Here's how the part is built. I have some questions about the finished solid (model axes, mm). Face numbers are marked on the shaded views. A direction names the side the tool comes from. Round coordinates to 2 decimals unless told otherwise and drop trailing zeros. Write each loop counter-clockwise with the first axis right and the second up, starting at its lowest first coordinate (ties: lowest second). Pieces come first, ordered by that corner, then holes. Notation, with made-up numbers: (12.5, 36.25) - (46.5, 36.25) arc R23 ccw to (46.5, 68.25) - close; hole circle Ø2 at (-25.75, 86.25). An arc over 180 degrees is marked (long way). Return JSON: item names as keys, results as strings. Group by question number.
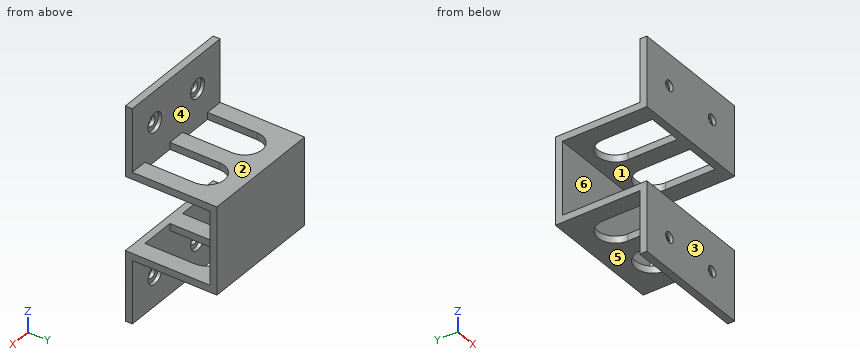
Autodesk Inventor part; units mm, degrees
ref_plane "YZ Plane" through (0, 0, 0) normal (1, 0, 0) x (0, 1, 0)
ref_plane "XZ Plane" through (0, 0, 0) normal (0, 1, 0) x (-1, 0, 0)
ref_plane "XY Plane" through (0, 0, 0) normal (0, 0, 1) x (1, 0, 0)
sketch "Sketch1" plane through (0, 0, 0) normal (0, 1, 0) x (-1, 0, 0)
  line L0 (0, 0) -> (-35, 0)
  line L1 (-35, 0) -> (-35, -20)
  line L2 (-35, -20) -> (0, -20)
  line L3 (0, -20) -> (0, 0)
  dimension "d0" = 35
  dimension "d1" = 20
extrude "Extrusion1" add sketch "Sketch1" along normal blind 2
sketch "Sketch2" plane through (0, 2, 0) normal (0, 1, 0) x (1, 0, 0)
  line L0 (0, 20) -> (0, 0)
  line L1 (35, 0) -> (35, 20)
  line L2 (0, 0) -> (35, 0)
  line L3 (35, 0) -> (35, 2)
  line L4 (35, 2) -> (0, 2)
  line L5 (0, 2) -> (0, 0)
  dimension "d4" = 2
extrude "Extrusion2" add sketch "Sketch2" along normal blind 24.2
sketch "Sketch3" plane through (0, 0, 0) normal (0, 0, 1) x (1, 0, 0)
  line L0 (0, 0) -> (0, 26.2)
  line L1 (35, 0) -> (35, 26.2)
  line L2 (0, 26.2) -> (35, 26.2)
  line L3 (35, 26.2) -> (35, 24.2)
  line L4 (35, 24.2) -> (0, 24.2)
  line L5 (0, 24.2) -> (0, 26.2)
  dimension "d7" = 2
extrude "Extrusion3" add sketch "Sketch3" along normal blind 23
sketch "Sketch4" plane through (0, 24.2, 0) normal (0, -1, 0) x (1, 0, 0)
  line L0 (35, -2) -> (35, 23)
  line L1 (0, 0) -> (0, 23)
  line L2 (35, 23) -> (0, 23)
  line L3 (0, 23) -> (0, 21)
  line L4 (0, 21) -> (35, 21)
  line L5 (35, 21) -> (35, 23)
  dimension "d10" = 2
extrude "Extrusion4" add sketch "Sketch4" along normal blind 24.2
sketch "Sketch5" plane through (0, 0, 23) normal (0, 0, 1) x (1, 0, 0)
  line L0 (0, 0) -> (0, 2)
  line L1 (35, 2) -> (0, 2)
  line L2 (0, 0) -> (35, 0)
  line L3 (35, 0) -> (35, 2)
  line L4 (35, 2) -> (0, 2)
  line L5 (0, 2) -> (0, 0)
extrude "Extrusion5" add sketch "Sketch5" along normal blind 18
sketch "Sketch6" plane through (0, 2, 0) normal (0, 1, 0) x (1, 0, 0)
  circle A0 centre (26, 11) radius 1.5
  line L0 (35, 20) -> (0, 20)
  line L1 (35, 2) -> (35, 20)
  circle A1 centre (9, 11) radius 1.5
  circle A2 centre (26, 11) radius 2.75
  circle A3 centre (9, 11) radius 2.75
  point P0 (0, 0)
  dimension "d15" = 3
  dimension "d16" = 9
  dimension "d17" = 9
  dimension "d18" = 3
  dimension "d19" = 17
  dimension "d20" = 5.5
  dimension "d21" = 5.5
extrude "Extrusion6" cut sketch "Sketch6" against normal blind 2 contours A0 | A1
extrude "Extrusion7" cut sketch "Sketch6" against normal blind 1
sketch "Sketch7" plane through (0, 2, 23) normal (0, 1, 0) x (1, 0, 0)
  circle A0 centre (26, -9) radius 1.5
  line L0 (35, -18) -> (0, -18)
  line L1 (35, 0) -> (35, -18)
  circle A1 centre (9, -9) radius 1.5
  circle A2 centre (26, -9) radius 2.75
  circle A3 centre (9, -9) radius 2.75
  point P0 (0, 23)
  dimension "d26" = 3
  dimension "d27" = 9
  dimension "d28" = 9
  dimension "d29" = 3
  dimension "d30" = 17
  dimension "d31" = 5.5
  dimension "d32" = 5.5
extrude "Extrusion8" cut sketch "Sketch7" against normal blind 2 contours A0 | A1
extrude "Extrusion9" cut sketch "Sketch7" against normal blind 1
sketch "Sketch8" plane through (35, 2, -2) normal (0, 0, -1) x (-1, 0, 0)
  arc A0 (15, 14.2) -> (5, 14.2) centre (10, 14.2) ccw
  line L0 (0, 24.2) -> (35, 24.2)
  line L1 (0, 0) -> (0, 24.2)
  line L2 (17.5, 24.2) -> (17.5, 0)
  line L3 (35, 0) -> (0, 0)
  line L4 (5, 14.2) -> (5, -0.3272)
  line L5 (15, 14.2) -> (15, 0)
  arc A1 (30, 14.2) -> (20, 14.2) centre (25, 14.2) ccw
  line L6 (30, 14.2) -> (30, -0.3272)
  line L7 (20, 14.2) -> (20, 0)
  point P0 (35, -2)
  point P1 (20, 0)
  point P2 (30, 0)
  point P3 (5, 0)
  dimension "d37" = 10
  dimension "d38" = 10
  dimension "d39" = 10
extrude "Extrusion10" cut sketch "Sketch8" against normal blind 25 contours L5 L3 L4 A0 | L7 A1 L6 L3
properties part number "Bracket Motor_3DPrint"
1) Will these pins go through, and if not, where does the flat tip stop? pin 1 Ø0.6 at (y, z) = (7, -1) entering from -X; pin 2 Ø1.6 at (x, z) = (8, -10) entering from +Y; pin 3 Ø4 at (x, z) = (30, 16) entering from -Y; pin 4 Ø12 at (x, y) = (19.5, 17) entering from -Z.
2) Imagine slicing it at D-D (x = 33.5). Please give me the cut outline in (y, z).
3) For the marked faces 1, 2 and 3, which set-ups out of +Z, -Z, +X, -X, +Y, -Y let a thin tool reach every point of the face, with its end or its side?
4) If we mould it in two halves opening along Z, with no side actions, what happens to the marked faces 4, 5 and 6? For each: released by +Z, released by -Z, zero draft, split by the parting line, or undercut.
5) I need wall thicknesses on line 1 along Z through (x, y) = (9, 1.4); line 2 along Z through (x, y) = (9, 0.4); line 3 along Y through (x, z) = (19, 1). Which ranges of each line are inside material? Lowest first, please.
6) Imagine slicing it at C-C (x = 26). Give the number of separate pieces and of enclosed holes in the cut face, plus the area to 3 significant figures.
7) Imagine slicing it at A-A (y = 14.5). Please give me the cut outline in (x, z), plus the area to 3 significant figures.
8) Imagine slicing it at B-B (z = -11). Please give me the cut outline in (x, y).
Results found:
{
 "1": {"pin 1": "stops at x = 0", "pin 2": "stops at y = 1", "pin 3": "stops at y = 24.2", "pin 4": "stops at z = -2"},
 "2": {"outline": "(0, -20) - (2, -20) - (2, -2) - (26.2, -2) - (26.2, 23) - (2, 23) - (2, 41) - (0, 41) - (0, 21) - (24.2, 21) - (24.2, 0) - (0, 0) - close"},
 "3": {"face 1": "+X, -X, -Y", "face 2": "+Z, +X, -X, +Y", "face 3": "+Z, -Z, +X, -X, -Y"},
 "4": {"face 4": "zero draft", "face 5": "released by -Z", "face 6": "undercut"},
 "5": {"line 1": "z = -20 to -13.75, -8.25 to 0, 21 to 29.25, 34.75 to 41", "line 2": "z = -20 to -12.5, -9.5 to 0, 21 to 30.5, 33.5 to 41", "line 3": "y = 24.2 to 26.2"},
 "6": {"separate pieces": "5", "enclosed holes": "0", "area": "125 mm²"},
 "7": {"outline": "(0, -2) - (5, -2) - (5, 0) - (0, 0) - close; (0, 21) - (5, 21) - (5, 23) - (0, 23) - close; (15, -2) - (20, -2) - (20, 0) - (15, 0) - close; (15, 21) - (20, 21) - (20, 23) - (15, 23) - close; (30, -2) - (35, -2) - (35, 0) - (30, 0) - close; (30, 21) - (35, 21) - (35, 23) - (30, 23) - close", "area": "60.0 mm²"},
 "8": {"outline": "(0, 0) - (7.5, 0) - (7.5, 1) - (6.25, 1) - (6.25, 2) - (0, 2) - close; (10.5, 0) - (24.5, 0) - (24.5, 1) - (23.25, 1) - (23.25, 2) - (11.75, 2) - (11.75, 1) - (10.5, 1) - close; (27.5, 0) - (35, 0) - (35, 2) - (28.75, 2) - (28.75, 1) - (27.5, 1) - close"}
}
